The figure shows three views and two pictorial views of one solid part (mm, origin at its lowest corner). Answer the questions. A direction names the side the tool comes from. Round coordinates to 2 decimals unless told otherwise and drop trailing zeros. Order: outer loops, then holes, each group sorted by start corner. A loop starts at its lowest first (then second) coordinate and runs counter-clockwise, first axis right, second up. Notation, with made-up numbers: M 83.5,-7.5 L 113.5,-7.5 A20 ccw 113.5,9.5 Z; hole C -1.5,24.5 d2. An arc over 180 degrees is marked long. Return JSON: item names as keys, results as strings.
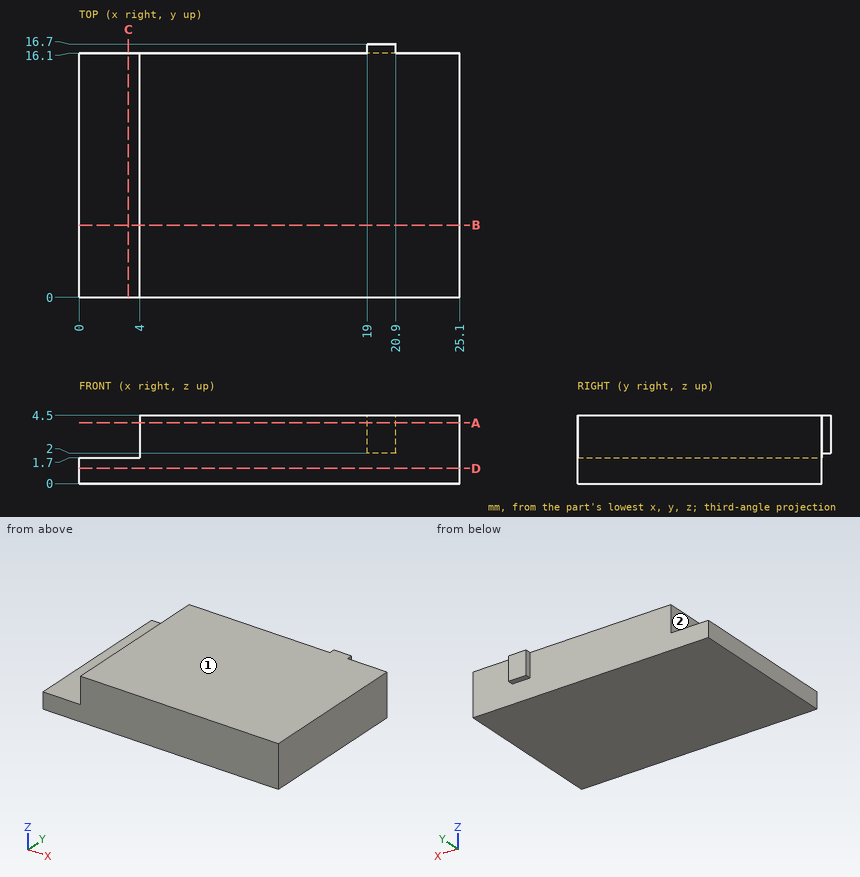
Item 1: Which of the six approach directions +Z, -Z, +X, -X, +Y, -Y give full straight-line access (tool end or side, diameter ignored) to the marked faces 1 and 2?
Output:
{"face 1": "+Z, +X, -X, +Y, -Y", "face 2": "+Z, -X, +Y, -Y"}
Item 2: Consider line 1 along Y through (x, z) = (16, 2.75); line 2 along X through (y, z) = (9.75, 2.7); line 3 along Z through (x, y) = (3, 7). Determine where each line is inside the solid, lowest interval first. Write a range as [from, to].
Output:
{"line 1": "y = [0, 16.1]", "line 2": "x = [4, 25.1]", "line 3": "z = [0, 1.7]"}
Item 3: Find section B-B (y = 4.75). Determine the outline of the cut face in (x, z), plus the area to 3 significant figures.
Output:
{"outline": "M 0,0 L 25.1,0 L 25.1,4.5 L 4,4.5 L 4,1.7 L 0,1.7 Z", "area": "102 mm^2"}
Item 4: Find section D-D (z = 1). Determine the outline of the cut face in (x, y), plus the area to 3 significant figures.
Output:
{"outline": "M 0,0 L 25.1,0 L 25.1,16.1 L 0,16.1 Z", "area": "404 mm^2"}
Item 5: Find section A-A (z = 4). Determine the outline of the cut face in (x, y), plus the area to 3 significant figures.
Output:
{"outline": "M 4,0 L 25.1,0 L 25.1,16.1 L 20.9,16.1 L 20.9,16.7 L 19,16.7 L 19,16.1 L 4,16.1 Z", "area": "341 mm^2"}
Item 6: Each of these flat-tipped pins is pushed along its axis until it touches: pin 1 (6 mm diameter, centred on x = 13.5, y = 3.5, fed in from -Z); pin 2 (0.5 mm diameter, centred on y = 16.5, z = 3, fed in from +X); pin 3 (0.8 mm diameter, centred on y = 7, z = 3.5, fed in from -X). Where does it stop, or does it pass through?
Output:
{"pin 1": "stops at z = 0", "pin 2": "stops at x = 20.9", "pin 3": "stops at x = 4"}
Item 7: Find section C-C (x = 3.25). Determine the outline of the cut face in (y, z).
Output:
{"outline": "M 0,0 L 16.1,0 L 16.1,1.7 L 0,1.7 Z"}
